from build123d import *

# Parameters (mm, degrees)
BOSS_EXTRUDE1_DEPTH = 5.334
CUT_EXTRUDE1_DEPTH  = 5.334
SKETCH6_R           = 1.5
SKETCH6_W           = 5.334
SKETCH6_H           = 4.572
CUT_EXTRUDE4_DEPTH  = 360.249845589
CUT_EXTRUDE5_DEPTH  = 360.249845589
CUT_EXTRUDE6_DEPTH  = 7.62
SKETCH11_W          = 12.7
SKETCH11_H          = 4.572
SKETCH11_W_2        = 4.572
SKETCH11_H_2        = 12.7
CUT_EXTRUDE9_DEPTH  = 360.249845589


with BuildPart() as part:
    # Sketch1 → Boss-Extrude1 (new body)
    with BuildSketch(Plane.XY):
        with BuildLine():
            Line((50.8, 0), (203.2, 0))
            ThreePointArc((203.2, 0), (239.121024484, 14.878975516), (254, 50.8))
            Line((254, 50.8), (254, 203.2))
            ThreePointArc((254, 203.2), (239.121024484, 239.121024484), (203.2, 254))
            Line((203.2, 254), (50.8, 254))
            ThreePointArc((50.8, 254), (14.878975516, 239.121024484), (0, 203.2))
            Line((0, 203.2), (0, 50.8))
            ThreePointArc((0, 50.8), (14.878975516, 14.878975516), (50.8, 0))
        make_face()
    extrude(amount=BOSS_EXTRUDE1_DEPTH)

    # Sketch3 → Cut-Extrude1 (cut)
    with BuildSketch(Plane.XY.offset(5.334)):
        Polygon((29.21, 95.25), (29.21, 88.9), (0, 88.9), (0, 165.1), (29.21, 165.1), (29.21, 158.75), (29.21, 146.05), (29.21, 133.35), (29.21, 120.65), (29.21, 107.95), align=None)
        Polygon((254, 165.1), (224.79, 165.1), (224.79, 158.75), (224.79, 146.05), (224.79, 133.35), (224.79, 120.65), (224.79, 107.95), (224.79, 95.25), (224.79, 88.9), (254, 88.9), align=None)
    extrude(amount=-CUT_EXTRUDE1_DEPTH, mode=Mode.SUBTRACT)

    # Sketch6 → Cut-Extrude4 (cut, through all)
    with BuildSketch(Plane.XY.offset(5.334)):
        with Locations((7.747, 185.928)):
            Circle(SKETCH6_R)
        with Locations(Location((246.253, 185.928, 0), (0, 0, 180))):
            Circle(SKETCH6_R)
        with Locations((246.253, 68.072)):
            Circle(SKETCH6_R)
        with Locations(Location((7.747, 68.072, 0), (0, 0, 180))):
            Circle(SKETCH6_R)
        with Locations((7.747, 194.564)):
            Rectangle(SKETCH6_W, SKETCH6_H)
        with Locations((7.747, 177.292)):
            Rectangle(SKETCH6_W, SKETCH6_H)
        with Locations((246.253, 177.292)):
            Rectangle(SKETCH6_W, SKETCH6_H)
        with Locations((246.253, 194.564)):
            Rectangle(SKETCH6_W, SKETCH6_H)
        with Locations((246.253, 59.436)):
            Rectangle(SKETCH6_W, SKETCH6_H)
        with Locations((246.253, 76.708)):
            Rectangle(SKETCH6_W, SKETCH6_H)
        with Locations((7.747, 76.708)):
            Rectangle(SKETCH6_W, SKETCH6_H)
        with Locations((7.747, 59.436)):
            Rectangle(SKETCH6_W, SKETCH6_H)
    extrude(amount=-CUT_EXTRUDE4_DEPTH, mode=Mode.SUBTRACT)

    # Sketch7 → Cut-Extrude5 (cut, through all)
    with BuildSketch(Plane.XY.offset(5.334)):
        with BuildLine():
            Line((78.555827904, 60.325), (78.555827904, 41.275))
            ThreePointArc((78.555827904, 41.275), (69.030827904, 31.75), (59.505827904, 41.275))
            Line((59.505827904, 41.275), (59.505827904, 60.325))
            ThreePointArc((59.505827904, 60.325), (69.030827904, 69.85), (78.555827904, 60.325))
        make_face()
        with BuildLine():
            Line((175.444172096, 60.325), (175.444172096, 41.275))
            ThreePointArc((175.444172096, 41.275), (184.969172096, 31.75), (194.494172096, 41.275))
            Line((194.494172096, 41.275), (194.494172096, 60.325))
            ThreePointArc((194.494172096, 60.325), (184.969172096, 69.85), (175.444172096, 60.325))
        make_face()
        with BuildLine():
            Line((175.444172096, 193.675), (175.444172096, 212.725))
            ThreePointArc((175.444172096, 212.725), (184.969172096, 222.25), (194.494172096, 212.725))
            Line((194.494172096, 212.725), (194.494172096, 193.675))
            ThreePointArc((194.494172096, 193.675), (184.969172096, 184.15), (175.444172096, 193.675))
        make_face()
        with BuildLine():
            Line((78.555827904, 193.675), (78.555827904, 212.725))
            ThreePointArc((78.555827904, 212.725), (69.030827904, 222.25), (59.505827904, 212.725))
            Line((59.505827904, 212.725), (59.505827904, 193.675))
            ThreePointArc((59.505827904, 193.675), (69.030827904, 184.15), (78.555827904, 193.675))
        make_face()
    extrude(amount=-CUT_EXTRUDE5_DEPTH, mode=Mode.SUBTRACT)

    # Sketch8 → Cut-Extrude6 (cut)
    with BuildSketch(Plane.XY.offset(5.334)):
        with BuildLine():
            Line((114.3, 69.85), (139.7, 69.85))
            ThreePointArc((139.7, 69.85), (146.05, 63.5), (139.7, 57.15))
            Line((139.7, 57.15), (114.3, 57.15))
            ThreePointArc((114.3, 57.15), (107.95, 63.5), (114.3, 69.85))
        make_face()
    extrude(amount=-CUT_EXTRUDE6_DEPTH, mode=Mode.SUBTRACT)

    # Sketch11 → Cut-Extrude9 (cut, through all)
    with BuildSketch(Plane.XY.offset(5.334)):
        Polygon((146.05, 182.372), (146.05, 177.8), (158.603579352, 177.8), (158.75, 177.8), (158.75, 182.372), align=None)
        with Locations((101.6, 180.086)):
            Rectangle(SKETCH11_W, SKETCH11_H)
        with Locations((199.136, 152.4)):
            Rectangle(SKETCH11_W_2, SKETCH11_H_2)
        Polygon((196.85, 108.5), (196.85, 107.95), (201.422, 107.95), (201.422, 120.65), (196.85, 120.65), align=None)
        with Locations((152.4, 86.614)):
            Rectangle(SKETCH11_W, SKETCH11_H)
        with Locations((101.6, 86.614)):
            Rectangle(SKETCH11_W, SKETCH11_H)
        with Locations((54.864, 114.3)):
            Rectangle(SKETCH11_W_2, SKETCH11_H_2)
        with Locations((54.864, 152.4)):
            Rectangle(SKETCH11_W_2, SKETCH11_H_2)
    extrude(amount=-CUT_EXTRUDE9_DEPTH, mode=Mode.SUBTRACT)


solid = part.part
The listing builds one solid part. Answer for the finished solid, in the listing's coordinates (mm). A direction names the side the tool comes from. Give positions to 0.01 mm unless a question says otherwise; leave off trailing zeros. Order: outer loops, then holes, each group sorted by start corner. A loop starts at its lowest first (then second) coordinate and runs counter-clockwise, first axis right, second up. Notation, with made-up numbers: (31.5, 76) - (72.5, 76) arc R13 cw to (72.5, 86) - close; hole circle Ø6 at (-24.5, 2). An arc over 180 degrees is marked (long way). One line per item, written item: value. Start each with the question number.
1) A cutting plane is placed at D-D on y = 17.5. Give the vertices of the cut face in (x, z).
2) A tool of negligible diameter and unlimited length cuts with its end or side. For faces 1 (the face through (15.276, 239.514, 2.63)), 2 (the face through (69.24, 222.248, 2.704)), from which of +Z, -Z, +X, -X, +Y, -Y can it reach the whole face along a straight path? Write none if from no direction.
3) A cutting plane is placed at C-C on z = 1.45. State how many separate pieces and enclosed holes the cut face has, then the cut area to 3 significant figures.
4) A cutting plane is placed at A-A on x = 128.5. Give the vertices of the cut face in (y, z), then the cut area to 3 significant figures.
5) Find the intervals of material crossed by L1, parallel to Y at x = 56, z = 2.25; L2, parallel to X at y = 193, z = 4.7; L3, parallel to X at y = 51, z = 2.15, in increasing order.
6) The mould has two halves that part along X. Classify faces 3 (the face through (125, 129, 0)), 4 (the face through (184.76, 31.752, 2.704)), 5 (the face through (14.486, 15.276, 2.63)): released by +X, released by -X, zero draft, split by the parting line, or undercut.
7) A cutting plane is placed at B-B on x = 18. Give the vertices of the cut face in (y, z).
8) Given pin 1 Ø3 at (y, z) = (148.5, 4) entering from +X; pin 2 Ø2.5 at (x, z) = (246, 3) entering from +Y; pin 3 Ø1.6 at (x, z) = (246, 2.5) entering from +Y, each flat-ended and moving along its own axis, determine where each tip first touches the part or whether it passes through.
Answer sheet:
1. outline: (12.44, 0) - (241.56, 0) - (241.56, 5.33) - (12.44, 5.33) - close
2. face 1: +Z, -Z, -X, +Y
2. face 2: +Z, -Z
3. separate pieces: 1
3. enclosed holes: 25
3. area: 54,100 mm2
4. outline: (0, 0) - (57.15, 0) - (57.15, 5.33) - (0, 5.33) - close; (69.85, 0) - (254, 0) - (254, 5.33) - (69.85, 5.33) - close
4. area: 1,290 mm2
5. L1: y = 0 to 107.95, 120.65 to 146.05, 158.75 to 254
5. L2: x = 0 to 5.08, 10.41 to 59.53, 78.53 to 175.47, 194.47 to 243.59, 248.92 to 254
5. L3: x = 0 to 59.51, 78.56 to 175.44, 194.49 to 254
6. face 3: zero draft
6. face 4: undercut
6. face 5: released by -X
7. outline: (12.01, 0) - (88.9, 0) - (88.9, 5.33) - (12.01, 5.33) - close; (165.1, 0) - (241.99, 0) - (241.99, 5.33) - (165.1, 5.33) - close
8. pin 1: stops at x = 224.79
8. pin 2: stops at y = 232.43
8. pin 3: stops at y = 231.78
